from build123d import *

# Parameters (mm, degrees)
PAD_DEPTH = 3


with BuildPart() as part:
    # Sketch (on XY_Plane of Origin) → Pad (new body)
    with BuildSketch(Plane.XY):
        with BuildLine():
            Line((-6, 4), (-6, -4))
            ThreePointArc((-6, -4), (-5.414214, -5.414214), (-4, -6))
            Line((-4, -6), (-1.75, -6))
            Line((-1.75, 2.083269), (-1.75, -6))
            ThreePointArc((-1.070312, 2.762957), (-1.550924, 2.563881), (-1.75, 2.083269))
            Line((1.070312, 2.762957), (-1.070312, 2.762957))
            ThreePointArc((1.75, 2.083269), (1.550924, 2.563881), (1.070312, 2.762957))
            Line((1.75, -6), (1.75, 2.083269))
            Line((1.75, -6), (4, -6))
            ThreePointArc((4, -6), (5.414214, -5.414214), (6, -4))
            Line((6, -4), (6, 4))
            ThreePointArc((6, 4), (5.414214, 5.414214), (4, 6))
            Line((4, 6), (-4, 6))
            ThreePointArc((-4, 6), (-5.414214, 5.414214), (-6, 4))
        make_face()
    extrude(amount=PAD_DEPTH)


solid = part.part
The listing builds one solid part. Answer for the finished solid, in the listing's coordinates (mm). A direction names the side the tool comes from. Coordinates: 2 decimals unless noted, no trailing zeros. Order: outer loops, then holes, each group sorted by start corner. A loop starts at its lowest first (then second) coordinate and runs counter-clockwise, first axis right, second up.
Q1. Which of the six approach directions +Z, -Z, +X, -X, +Y, -Y give full straight-line access (tool end or side, diameter ignored) to faces 4 (the face through (1.75, -2, 1)), 5 (the face through (-5.4, 5.43, 1.48))?
Q2. A cutting plane is placed at B-B, the plane z = 1.05. Write down the section's boundary in (x, y), and give its area (3 significant figures).
Q3. A cutting plane is placed at A-A, the plane y = 1. Write down the section's boundary in (x, z).
Q4. For a pull along X with two mould halves and no side action, classify faces 1 (the face through (5.4, -5.43, 1.48)), 2 (the face through (-1.75, -2, 1)), 3 (the face through (-6, 0, 1)) as pulls with the +X half, pulls with the -X half, needs draft (parallel to the pull), parting line crosses it, or undercut.
Q5. Consider line 1 (X direction, y = -3.75, z = 0.1); line 2 (Y direction, x = -1, z = 1.9); line 3 (X direction, y = 2.5, z = 1.25). Determine where each line is inside the solid, lowest interval first.
Q6. A cutting plane is placed at C-C, the plane x = -5. Write down the section's boundary in (y, z).
Q7. Given P1, Ø1.5, axis at x = 2, y = 4, coming from the -Z side; P2, Ø1, axis at x = 1, y = -2.5, coming from the +Z side, each flat-ended and moving along its own axis, determine where each tip first touches the part or whether it passes through.
Answers follow:
1. face 4: +Z, -Z, -Y
1. face 5: +Z, -Z, -X, +Y
2. outline: (-6, -4) arc R2 ccw to (-4, -6) - (-1.75, -6) - (-1.75, 2.08) arc R0.68 cw to (-1.07, 2.76) - (1.07, 2.76) arc R0.68 cw to (1.75, 2.08) - (1.75, -6) - (4, -6) arc R2 ccw to (6, -4) - (6, 4) arc R2 ccw to (4, 6) - (-4, 6) arc R2 ccw to (-6, 4) - close
2. area: 110 mm2
3. outline: (-6, 0) - (-1.75, 0) - (-1.75, 3) - (-6, 3) - close; (1.75, 0) - (6, 0) - (6, 3) - (1.75, 3) - close
4. face 1: pulls with the +X half
4. face 2: undercut
4. face 3: pulls with the -X half
5. line 1: x = -6 to -1.75, 1.75 to 6
5. line 2: y = 2.76 to 6
5. line 3: x = -6 to -1.61, 1.61 to 6
6. outline: (-5.73, 0) - (5.73, 0) - (5.73, 3) - (-5.73, 3) - close
7. P1: stops at z = 0
7. P2: passes through
